The model under review builds one solid part; all positions refer to its coordinate system, in mm. Face numbers are marked on the shaded views. A direction names the side the tool comes from. Round coordinates to 2 decimals unless told otherwise and drop trailing zeros. Order: outer loops, then holes, each group sorted by start corner. A loop starts at its lowest first (then second) coordinate and runs counter-clockwise, first axis right, second up.
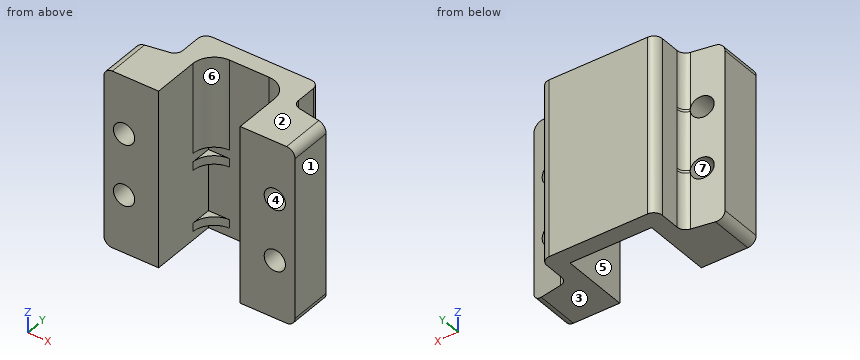
from build123d import *

# Parameters (mm, degrees)
BOSS_EXTRUDE1_DEPTH      = 3.556
BOSS_EXTRUDE1_DEPTH_BACK = 22.86
BOSS_EXTRUDE2_DEPTH      = 13.462
BOSS_EXTRUDE3_START      = -1.27
BOSS_EXTRUDE3_DEPTH      = 1.905
FILLET1_R                = 1.27
BOSS_EXTRUDE4_DEPTH      = 8.509
CUT_EXTRUDE1_DEPTH       = 7.874


with BuildPart() as part:
    # Sketch1 → Boss-Extrude1 (new body, two sides)
    with BuildSketch(Plane.XY) as boss_extrude1_sk:
        Polygon((-6.096, 10.16), (6.096, 10.16), (6.096, 0), (14.2875, 0), (14.2875, 6.35), (8.636, 7.346511931), (8.636, 12.7), (-8.636, 12.7), (-8.636, 7.346511931), (-14.2875, 6.35), (-14.2875, 0), (-6.096, 0), align=None)
    extrude(amount=BOSS_EXTRUDE1_DEPTH)
    extrude(boss_extrude1_sk.sketch, amount=-BOSS_EXTRUDE1_DEPTH_BACK)

    # Sketch2 → Boss-Extrude2 (add)
    with BuildSketch(Plane.XY.offset(3.556)):
        with BuildLine():
            Line((2.921, 10.16), (6.096, 10.16))
            Line((6.096, 10.16), (6.096, 6.985))
            ThreePointArc((6.096, 6.985), (5.16606403, 9.23006403), (2.921, 10.16))
        make_face()
        with BuildLine():
            Line((-6.096, 10.16), (-6.096, 6.985))
            ThreePointArc((-6.096, 6.985), (-5.16606403, 9.23006403), (-2.921, 10.16))
            Line((-2.921, 10.16), (-6.096, 10.16))
        make_face()
    extrude(amount=-BOSS_EXTRUDE2_DEPTH)

    # Sketch3 → Boss-Extrude3 (add)
    with BuildSketch(Plane.XY.offset(-9.906).offset(BOSS_EXTRUDE3_START)):
        with BuildLine():
            Line((-6.096, 10.16), (-6.096, 6.985))
            ThreePointArc((-6.096, 6.985), (-5.16606403, 9.23006403), (-2.921, 10.16))
            Line((-2.921, 10.16), (-6.096, 10.16))
        make_face()
    extrude(amount=-BOSS_EXTRUDE3_DEPTH)

    # Sketch6 → Cut-Revolve1 (revolve, cut)
    with BuildSketch(Plane.XY.offset(-5.08)):
        Polygon((11.262482277, -1.27), (12.849982277, -1.27), (12.849982277, 6.60347316), (12.849982277, 9.423392242), (11.262482277, 9.423392242), (11.262482277, 6.883392242), align=None)
    cut_revolve1 = revolve(axis=Axis((11.262482277, -1.27, -5.08), (0, -1, 0)), mode=Mode.SUBTRACT)

    # Mirror1: Cut-Revolve1 across plane
    add(cut_revolve1.mirror(Plane(origin=(0, 0, 0), x_dir=(0, 0, 1), z_dir=(1, 0, 0))), mode=Mode.SUBTRACT)

    # Mirror2: Cut-Revolve1 across plane
    add(cut_revolve1.mirror(Plane.XY.offset(-9.652)), mode=Mode.SUBTRACT)

    # Mirror2 copy 1 sketch → Mirror2 copy 1 (revolve, cut)
    with BuildSketch(Plane(origin=(0, 0, -14.224), x_dir=(-1, 0, 0), z_dir=(0, 0, -1))):
        Polygon((11.262482277, -1.27), (12.849982277, -1.27), (12.849982277, 6.60347316), (12.849982277, 9.423392242), (11.262482277, 9.423392242), (11.262482277, 6.883392242), align=None)
    revolve(axis=Axis((-11.262482277, -1.27, -14.224), (0, -1, 0)), mode=Mode.SUBTRACT)

    # Fillet1
    fillet1_edges = [part.edges().sort_by_distance(p)[0] for p in [
        (14.2875, 3.175, 3.556),
        (-8.636, 7.346511931, -9.652),
        (-8.636, 12.7, -9.652),
        (8.636, 12.7, -9.652),
        (8.636, 7.346511931, -9.652),
        (-14.2875, 3.175, -22.86),
        (14.2875, 3.175, -22.86),
        (-14.2875, 3.175, 3.556),
    ]]
    fillet(fillet1_edges, radius=FILLET1_R)

    # Sketch4 → Boss-Extrude4 (add)
    with BuildSketch(Plane.XY.offset(-13.081)):
        with BuildLine():
            Line((-6.096, 10.16), (-6.096, 6.985))
            ThreePointArc((-6.096, 6.985), (-5.16606403, 9.23006403), (-2.921, 10.16))
            Line((-2.921, 10.16), (-6.096, 10.16))
        make_face()
    extrude(amount=-BOSS_EXTRUDE4_DEPTH)

    # Sketch9 → Cut-Extrude1 (cut)
    with BuildSketch(Plane.XY.offset(-12.446)):
        Polygon((-6.096, 6.985), (-5.987323019, 7.808582504), (-5.675836906, 8.563448168), (-5.16606403, 9.23006403), (-4.513044207, 9.732002047), (-3.747031782, 10.05066412), (-2.921, 10.16), (-6.096, 10.16), align=None)
    extrude(amount=-CUT_EXTRUDE1_DEPTH, mode=Mode.SUBTRACT)


solid = part.part
(1) We need section C-C (y = 2.5). Give the boundary of the cut face in (x, z) (1 decimal).
(2) We need section B-B (z = -19.5). Give the boundary of the cut face in (x, y).
(3) To check wall thickness, follow L1, parallel to X at y = 4, z = -5.08; L2, parallel to X at y = 5.75, z = -18.25; L3, parallel to X at y = 10, z = -18.5. State the ranges of each line that lie inside material, in increasing order.
(4) The part is to be moulded in two halves that separate along Z. For the marked faces 1, 2, 3 and 4, say which applies: pulls with the +Z half, pulls with the -Z half, needs draft (parallel to the pull), parting line crosses it, or undercut.
(5) We need section A-A (y = 9.5). Give the boundary of the cut face in (x, z).
(6) Clearance check with flat-ended pins moving along their axes: P1, Ø1, axis at x = 4.5, y = 9, coming from the -Z side; P2, Ø2, axis at x = 9, z = -19.5, coming from the +Y side; P3, Ø1.5, axis at y = 10.5, z = -6, coming from the +X side; P4, Ø2.5, axis at y = 9.5, z = -5.5, coming from the -X side. State where each tip first meets the part, or that it passes through.
(7) Tool access review of the marked faces 5, 6 and 7: name each direction out of +Z, -Z, +X, -X, +Y, -Y from which nothing blocks a thin tool from reaching the whole face with its end or side.
Verdict:
1. outline: (-14.3, -21.6) arc R1.3 ccw to (-13, -22.9) - (-6.1, -22.9) - (-6.1, 3.6) - (-13, 3.6) arc R1.3 ccw to (-14.3, 2.3) - close; (6.1, -22.9) - (13, -22.9) arc R1.3 ccw to (14.3, -21.6) - (14.3, 2.3) arc R1.3 ccw to (13, 3.6) - (6.1, 3.6) - close; hole circle Ø3.2 at (-11.3, -14.2); hole circle Ø3.2 at (-11.3, -5.1); hole circle Ø3.2 at (11.3, -14.2); hole circle Ø3.2 at (11.3, -5.1)
2. outline: (-14.29, 0) - (-6.1, 0) - (-6.1, 10.16) - (6.1, 10.16) - (6.1, 0) - (14.29, 0) - (14.29, 6.35) - (9.69, 7.16) arc R1.27 cw to (8.64, 8.41) - (8.64, 11.43) arc R1.27 ccw to (7.37, 12.7) - (-7.37, 12.7) arc R1.27 ccw to (-8.64, 11.43) - (-8.64, 8.41) arc R1.27 cw to (-9.69, 7.16) - (-14.29, 6.35) - close
3. L1: x = -14.29 to -12.85, -9.67 to -6.1, 6.1 to 9.67, 12.85 to 14.29
3. L2: x = -14.29 to -6.1, 6.1 to 14.29
3. L3: x = -8.64 to -6.1, 6.1 to 8.64
4. face 1: needs draft
4. face 2: pulls with the +Z half
4. face 3: pulls with the -Z half
4. face 4: undercut
5. outline: (-8.64, -22.86) - (-6.1, -22.86) - (-6.1, -21.59) - (-4.86, -21.59) - (-4.86, -20.32) - (-6.1, -20.32) - (-6.1, -12.45) - (-4.86, -12.45) - (-4.86, -11.18) - (-6.1, -11.18) - (-6.1, -9.91) - (-4.86, -9.91) - (-4.86, 3.56) - (-8.64, 3.56) - close; (4.86, -9.91) - (6.1, -9.91) - (6.1, -22.86) - (8.64, -22.86) - (8.64, 3.56) - (4.86, 3.56) - close
6. P1: passes through
6. P2: stops at y = 12.53
6. P3: stops at x = 8.64
6. P4: stops at x = -8.65
7. face 5: -Z, -Y
7. face 6: +Z, -Z, -Y
7. face 7: +Y, -Y
